Autodesk Inventor part; units mm, degrees
ref_plane "Work Plane1" through (29, 0, 0) normal (0, -1, 0) x (1, 0, 0)
ref_plane "YZ Plane" through (0, 0, 0) normal (1, 0, 0) x (0, 1, 0)
ref_plane "XZ Plane" through (0, 0, 0) normal (0, 1, 0) x (-1, 0, 0)
sketch "Sketch1" plane through (0, 0, 0) normal (0, 0, 1) x (1, 0, 0)
  line L0 (-0.6667, 0) -> (60, 0)
  line L1 (60, 0) -> (60, 1.5)
  line L2 (60, 1.5) -> (42, 1.5)
  line L3 (42, 1.5) -> (41.6932, 1.5)
  line L4 (41.6932, 1.5) -> (0, 1.5)
  line L5 (0, 1.5) -> (0, 2.75)
  line L6 (0, 2.75) -> (-3, 2.75)
  line L7 (-3, 2.75) -> (-3, 1.4434)
  line L8 (-3, 1.4434) -> (-1.5, 1.4434)
  line L9 (-1.5, 1.4434) -> (-0.6667, 0)
  line L10 (-15.6, 0) -> (72.6, 0)
  line L11 (0, -0.55) -> (0, 3.3)
  line L12 (42, 1.5) -> (0, 1.5) construction
  dimension "d1" = 18
  dimension "d2" = 0.3068
  dimension "d3" = 3
  dimension "d4" = 1.5
  dimension "d5" = 60
  dimension "d6" = 3
  dimension "d7" = 3
  dimension "d8" = 2.8868
  dimension "d9" = 5.5
  dimension "d26" = 60
revolve "Body" add sketch "Sketch1" angle 360 about axis through (-0.6667, 0, 0) along (1, 0, 0)
sketch "Sketch2" plane through (-3, 0, 0) normal (-1, 0, 0) x (0, 0, 1)
  circle A0 centre (0, 0) radius 1.4434
  line L0 (0, -3.85) -> (0, 3.85)
  line L1 (-3.85, 0) -> (3.85, 0)
  line L2 (1.4434, 0) -> (0.7217, -1.25)
  line L3 (0.7217, -1.25) -> (-0.7217, -1.25)
  line L4 (-0.7217, -1.25) -> (-1.4434, 0)
  line L5 (-1.4434, 0) -> (-0.7217, 1.25)
  line L6 (-0.7217, 1.25) -> (0.7217, 1.25)
  line L7 (0.7217, 1.25) -> (1.4434, 0)
  point P0 (0, 0)
extrude "Slot" add sketch "Sketch2" against normal up to next contours L7 A0 | A0 L2 | L6 L0 A0 | A0 L0 L3 | L0 L6 A0 | A0 L3 L0 | L4 A0 | A0 L5
fillet "Fillet1" radius 0.3 1 edges at (-3, -2.75, 0)
thread "Thread"
chamfer "Chamfer1" distance 0.3067 distance2 0.3067 1 edges at (60, -1.5, 0) measured on face at (60, -0.3743, 0.3316)
ref_plane "Work Plane1" through (29, 0, 0) normal (0, -1, 0) x (1, 0, 0)
fillet "Fillet2" radius 0.1 1 edges at (0, -1.5, 0)
equation "\"d1\" = GEL"
equation "\"d3\" = KOH"
equation "\"d4\" = INTI"
equation "\"d6\" = GD"
equation "\"d7\" = BDM"
equation "\"d8\" = 1.1547 * SW"
equation "\"d9\" = KOD"
equation "\"d26\" = NLG"
equation "\"d30\" = R"
equation "\"d17\" = RR"
equation "\"d13\" = GEL"
equation "\"d15\" = -0.5 * SPD + 0.5 * GD"
equation "\"d16\" = GUL"
equation "\"GD\" = NND"
equation "\"NLG\" = 60"
equation "\"GEL\" = 18"
equation "\"KOD\" = 5.5"
equation "\"KOH\" = 3"
equation "\"INTI\" = 1.5"
equation "\"GAL\" = 0.61345 * PTC"
equation "\"GUL\" = 0.61345 * PTC"
equation "\"BDM\" = NND"
equation "\"SW\" = 2.5"
equation "\"RR\" = 0.3"
equation "\"SPD\" = 2.38655"
equation "\"R\" = 0.1"
equation "\"TOA\" = 30deg"
equation "\"THREADDIA\" = 3"
equation "\"PTC\" = 0.5"
equation "\"NND\" = 3"
equation "\"E0\" = 1.155 * SW"
equation "\"GD1\" = THREADDIA - 1.2269 * PTC"
properties part number "ANSI B18.3.1M - M3x0.5 x 60" material "Steel, Mild"
Can you work these out from the model? Positions are in its coordinate system, mm. A direction names the side the tool comes from. Coordinates: 2 decimals unless noted, no trailing zeros. Loops run counter-clockwise (first coordinate to the right, second up) from the corner with the lowest first, then second, coordinate; pieces in that order, holes last.
1) For pin 1 (1 mm diameter, centred on x = 19.5, y = -1.5, fed in from +Z); pin 2 (3 mm diameter, centred on x = 52, z = -2, fed in from +Y), each with a flat end and sliding along its axis, tell me the tip position at first contact or that it passes through.
2) Thinking about a two-plate mould opening in Y: for faces 4 (the cylindrical face through (-1.369, -0.596, 2.685)), 5 (the flat face through (-2.205, 0.616, -1.088)), 6 (the flat face through (0, 2, 0)), which applies, pulls with the +Y half, pulls with the -Y half, needs draft (parallel to the pull), parting line crosses it, or undercut?
3) I need wall thicknesses on probe 1 along Z at (x, y) = (29, 0.2); probe 2 along X at (y, z) = (-0.15, 1.9). Which ranges of each line are inside material? Lowest first, please.
4) Imagine slicing it at A-A on x = 22. List the corners of the cut face in (y, z) for me, plus the area to 3 significant figures.
5) Which directions (+Z, -Z, +X, -X, +Y, -Y) give clear straight access to the entire face, cutting with the end or side of a thin tool? Please do faces 1 (the cylindrical face through (29.48, -1.5, -0.07)), 2 (the flat face through (-2, 1.25, 0)), 3 (the flat face through (-3, -1.1, 1.1)).
Completed:
1. pin 1: stops at z = 1.12
1. pin 2: stops at y = 1.41
2. face 4: parting line crosses it
2. face 5: undercut
2. face 6: needs draft
3. probe 1: z = -1.49 to 1.49
3. probe 2: x = -3 to 0
4. outline: circle Ø3 at (0, 0)
4. area: 7.07 mm2
5. face 1: +X
5. face 2: -X
5. face 3: +Z, -Z, -X, +Y, -Y
